```python
from build123d import *

# Parameters (mm, degrees)
SKETCH4_R           = 3.683
BOSS_EXTRUDE1_DEPTH = 5.789022458
SKETCH5_R           = 5.08
BOSS_EXTRUDE2_DEPTH = 2.54


with BuildPart() as part:
    # Sketch2 → Revolve1 (revolve)
    with BuildSketch(Plane.XY, mode=Mode.PRIVATE) as revolve1_sk:
        with BuildLine():
            Line((-18.415, 0), (-18.415, 15.697572511))
            ThreePointArc((-18.415, 15.697572511), (-9.266184884, 17.257739329), (0, 17.78))
            ThreePointArc((0, 17.78), (9.266184884, 17.257739329), (18.415, 15.697572511))
            Line((18.415, 15.697572511), (18.415, 0))
            Line((18.415, 0), (-18.415, 0))
        make_face()
    revolve(revolve1_sk.sketch.rotate(Axis((-18.415, 0, 0), (1, 0, 0)), 90), axis=Axis((-18.415, 0, 0), (1, 0, 0)))

    # Sketch4 → Boss-Extrude1 (add)
    with BuildSketch(Plane(origin=(18.415, 0, 0), x_dir=(0, 0, -1), z_dir=(1, 0, 0))):
        Circle(SKETCH4_R)
    boss_extrude1 = extrude(amount=BOSS_EXTRUDE1_DEPTH)

    # Sketch5 → Boss-Extrude2 (add)
    with BuildSketch(Plane(origin=(24.204022458, 0, 0), x_dir=(0, 0, -1), z_dir=(1, 0, 0))):
        Circle(SKETCH5_R)
    boss_extrude2 = extrude(amount=BOSS_EXTRUDE2_DEPTH)

    # Mirror1: Boss-Extrude1, Boss-Extrude2 across plane
    add(boss_extrude1.mirror(Plane(origin=(0, 0, 0), x_dir=(0, 0, 1), z_dir=(1, 0, 0))))
    add(boss_extrude2.mirror(Plane(origin=(0, 0, 0), x_dir=(0, 0, 1), z_dir=(1, 0, 0))))


solid = part.part
```
Can you work these out from the model? Positions are in its coordinate system, mm. A direction names the side the tool comes from. Give positions to 0.01 mm unless a question says otherwise; leave off trailing zeros. Write each loop counter-clockwise with the first axis right and the second up, starting at its lowest first coordinate (ties: lowest second). Pieces come first, ordered by that corner, then holes. Notation, with made-up numbers: (-19, -17.75) -> (5, -17.75) arc R29 cw to (5, 13.25) -> close; hole circle Ø4 at (32.5, -37). An arc over 180 degrees is marked (long way). Write item = value, one per line.
(1) For faces 1 (the face through (-26.744, 0, 0)), 2 (the face through (26.744, 0, 0)), 3 (the face through (-25.456, 5.037, 0.661)), 4 (the face through (-24.204, 3, -3)), 5 (the face through (25.456, 5.037, 0.661)), which set-ups out of +Z, -Z, +X, -X, +Y, -Y let a thin tool reach every point of the face, with its end or its side?
Worked out:
face_1 = +Z, -Z, -X, +Y, -Y
face_2 = +Z, -Z, +X, +Y, -Y
face_3 = -X
face_4 = none
face_5 = +X
(2) I'm going to push flat-ended pins straight in: P1, Ø4, axis at y = -4.5, z = 11.5, coming from the -X side (3 decimals); P2, Ø12, axis at x = 9.5, y = 3, coming from the -Z side; P3, Ø8, axis at y = 8, z = 13.5, coming from the +X side (3 decimals). Where does each tip first touch, or does it pass through?
Worked out:
P1 = -18.415
P2 = -17.67
P3 = 18.415
(3) I need wall thicknesses on probe 1 along X at (y, z) = (-8, 3) (3 decimals); probe 2 along Y at (x, z) = (24.5, -2); probe 3 along Z at (x, y) = (-13, 14.5). Which ranges of each line are inside material? Lowest first, please. Write a range as from..to.
Worked out:
probe_1 = -18.415..18.415
probe_2 = -4.67..4.67
probe_3 = -8.38..8.38
(4) Suppose I cut it at A-A on x = 23. Write out the boundary of the cut face in (y, z).
Worked out:
outline = circle Ø7.37 at (0, 0)
